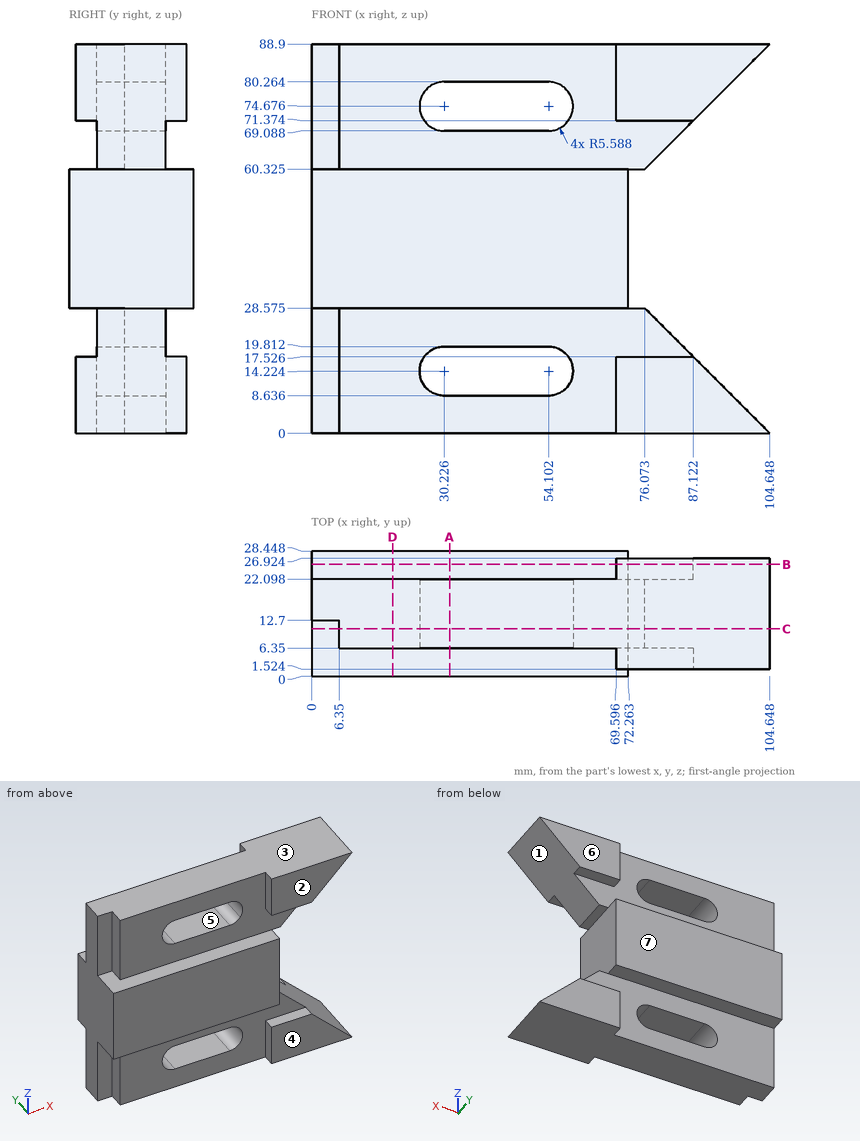
Verification items for this drawing (mm, ordinates from the low corner). A direction names the side the tool comes from. Give positions to 0.01 mm unless a question says otherwise; leave off trailing zeros. Write each loop counter-clockwise with the first axis right and the second up, starting at its lowest first coordinate (ties: lowest second). Pieces come first, ordered by that corner, then holes. Notation, with made-up numbers: (38.5, 20.5) - (72.5, 20.5) arc R19 cw to (72.5, 29.5) - close; hole circle Ø4 at (-40, 32.5). An arc over 180 degrees is marked (long way). Answer as CSV lines item,"result". Start each with the question number.
1. Sectioned sample at A-A (x = 31.5). Record the boundary of the cut face in (y, z) (3 decimals), then the cut area to 3 significant figures.
2. Thickness scan on line 1 (Z direction, x = 29, y = 19.5); line 2 (Y direction, x = 70, z = 5); line 3 (Y direction, x = 19, z = 21.5). Record the ranges inside material, lowest first.
3. Sectioned sample at C-C (y = 10.75). Record the boundary of the cut face in (x, z) (3 decimals).
4. Depth check by flat-ended pin: pin 1 (6 mm diameter, centred on x = 63, z = 19.5, fed in from +Y); pin 2 (23 mm diameter, centred on x = 59.5, z = 75, fed in from -Y); pin 3 (1.5 mm diameter, centred on x = 59.5, z = 68, fed in from -Y). Enter the tip coordinate at first touch or a pass-through.
5. Set-up check for the marked faces 4, 5, 6 and 7: record each of +Z, -Z, +X, -X, +Y, -Y from which the full face is reachable in a straight line by a thin tool's end or side.
6. Draft check along Z on the marked faces 1, 2 and 3. Enter one of: pulls with the +Z half, pulls with the -Z half, needs draft (parallel to the pull), parting line crosses it, or undercut.
7. Sectioned sample at B-B (y = 25.5). Record the boundary of the cut face in (x, z) (3 decimals), then the cut area to 3 significant figures.
8. Sectioned sample at D-D (x = 18.5). Record the boundary of the cut face in (y, z) (3 decimals).
Derived:
1,outline,"(0, 28.575) - (6.35, 28.575) - (6.35, 19.812) - (22.098, 19.812) - (22.098, 28.575) - (28.448, 28.575) - (28.448, 60.325) - (22.098, 60.325) - (22.098, 69.088) - (6.35, 69.088) - (6.35, 60.325) - (0, 60.325) - close; (6.35, 0) - (22.098, 0) - (22.098, 8.636) - (6.35, 8.636) - close; (6.35, 80.264) - (22.098, 80.264) - (22.098, 88.9) - (6.35, 88.9) - close"
1,area,"1,450 mm²"
2,line 1,"0 to 8.77, 19.68 to 69.22, 80.13 to 88.9"
2,line 2,"1.52 to 26.92"
2,line 3,"6.35 to 22.1"
3,outline,"(0, 28.575) - (6.35, 28.575) - (6.35, 0) - (104.648, 0) - (76.073, 28.575) - (72.263, 28.575) - (72.263, 60.325) - (76.073, 60.325) - (104.648, 88.9) - (6.35, 88.9) - (6.35, 60.325) - (0, 60.325) - close; hole (30.226, 8.636) - (54.102, 8.636) arc R5.588 ccw to (54.102, 19.812) - (30.226, 19.812) arc R5.588 ccw to start; hole (30.226, 69.088) - (54.102, 69.088) arc R5.588 ccw to (54.102, 80.264) - (30.226, 80.264) arc R5.588 ccw to start"
4,pin 1,"y = 22.1"
4,pin 2,"y = 1.52"
4,pin 3,"y = 6.35"
5,face 4,"-Z, +X, -X, -Y"
5,face 5,"+Y, -Y"
5,face 6,"+Z, +X, -X, +Y"
5,face 7,"+Z, -Z, +X, -X, +Y"
6,face 1,"undercut"
6,face 2,"needs draft"
6,face 3,"pulls with the +Z half"
7,outline,"(0, 28.575) - (72.263, 28.575) - (72.263, 60.325) - (0, 60.325) - close; (69.596, 0) - (104.648, 0) - (87.122, 17.526) - (69.596, 17.526) - close; (69.596, 71.374) - (87.122, 71.374) - (104.648, 88.9) - (69.596, 88.9) - close"
7,area,"3,220 mm²"
8,outline,"(0, 28.575) - (6.35, 28.575) - (6.35, 0) - (22.098, 0) - (22.098, 28.575) - (28.448, 28.575) - (28.448, 60.325) - (22.098, 60.325) - (22.098, 88.9) - (6.35, 88.9) - (6.35, 60.325) - (0, 60.325) - close"
